Build history of the part. All positions in model axes, mm. A direction names the side the tool comes from. Coordinates: 2 decimals unless noted, no trailing zeros. Order: outer loops, then holes, each group sorted by start corner. A loop starts at its lowest first (then second) coordinate and runs counter-clockwise, first axis right, second up. Notation, with made-up numbers: (-33.75, 41) - (-27.75, 41) arc R17 cw to (-27.75, 62) - close; hole circle Ø9 at (-4.75, -8.5). An arc over 180 degrees is marked (long way). Write each question's results on one line, items separated by ' | '.
from build123d import *

# Parameters (mm, degrees)
SKETCH2_R           = 4.25
SKETCH2_R_2         = 4
BOSS_EXTRUDE1_DEPTH = 15
FILLET1_R           = 1.5


with BuildPart() as part:
    # Sketch2 → Boss-Extrude1 (new body)
    with BuildSketch(Plane.XY):
        with BuildLine():
            Line((0, -35), (26, -35))
            Line((26, -35), (26, -25))
            Line((26, -25), (18, -25))
            Line((18, -25), (18, 0))
            Line((18, 0), (0, 0))
            Line((0, 0), (-18.303795088, -24.696911327))
            Line((-18.303795088, -24.696911327), (-28.121591697, -31.596974351))
            ThreePointArc((-28.121591697, -31.596974351), (-29.945175188, -42.045636622), (-19.496512917, -43.869220113))
            Line((-19.496512917, -43.869220113), (-9.678716308, -36.969157088))
            Line((-9.678716308, -36.969157088), (0, -35))
        make_face()
        with Locations((9, -12.5)):
            Circle(SKETCH2_R, mode=Mode.SUBTRACT)
        with Locations((-23.809052307, -37.733097232)):
            Circle(SKETCH2_R_2, mode=Mode.SUBTRACT)
    extrude(amount=BOSS_EXTRUDE1_DEPTH)

    # Fillet1
    fillet1_edges = [part.edges().sort_by_distance(p)[0] for p in [
        (0, 0, 7.5),
    ]]
    fillet(fillet1_edges, radius=FILLET1_R)


solid = part.part
1. Band-saw the part on C-C on z = 10.5. Give the cut face in (x, y), then the cut area to 3 significant figures.
Solved:
outline: (-28.12, -31.6) arc R7.5 ccw to (-19.5, -43.87) - (-9.68, -36.97) - (0, -35) - (26, -35) - (26, -25) - (18, -25) - (18, 0) - (0.76, 0) arc R1.5 ccw to (-0.45, -0.61) - (-18.3, -24.7) - close; hole circle Ø8 at (-23.81, -37.73); hole circle Ø8.5 at (9, -12.5) | area: 1,260 mm2
2. Two-plate mould, pull along X, no slides. Class faces 4 (the face through (18, -13, 7)), 5 (the face through (-24.676, -41.638, 7.395)), 6 (the face through (5.63, -15.09, 7.4)), 7 (the face through (0.089, -0.156, 7.605)): +X half, -X half, draft (parallel to the pull), parting line (faces both ways), or undercut.
Solved:
face 4: +X half | face 5: undercut | face 6: undercut | face 7: -X half
3. Probe line 1 (Y direction, x = 9, z = 9.25); line 2 (Y direction, x = -23, z = 7.75); line 3 (Y direction, x = 22, z = 5.5). List the from-to ranges inside material, lowest first.
Solved:
line 1: y = -35 to -16.75, -8.25 to 0 | line 2: y = -45.19 to -41.65, -33.82 to -28 | line 3: y = -35 to -25
4. Band-saw the part on D-D on x = 21. Give the cut face in (y, z).
Solved:
outline: (-35, 0) - (-25, 0) - (-25, 15) - (-35, 15) - close
5. Band-saw the part on B-B on y = -41. Give the cut face in (x, z).
Solved:
outline: (-30.56, 0) - (-26.12, 0) - (-26.12, 15) - (-30.56, 15) - close; (-21.5, 0) - (-15.41, 0) - (-15.41, 15) - (-21.5, 15) - close
6. Band-saw the part on A-A on x = 9. Give the cut face in (y, z), then the cut area to 4 significant figures.
Solved:
outline: (-35, 0) - (-16.75, 0) - (-16.75, 15) - (-35, 15) - close; (-8.25, 0) - (0, 0) - (0, 15) - (-8.25, 15) - close | area: 397.5 mm2
7. Tool access for faces 1 (the face through (22, -25, 7)), 2 (the face through (9, 0, 7)), 3 (the face through (13, -35, 7)): list every direction of +Z, -Z, +X, -X, +Y, -Y with a clear straight run to the whole face (end or side of a thin tool).
Solved:
face 1: +Z, -Z, +X, +Y | face 2: +Z, -Z, +X, -X, +Y | face 3: +Z, -Z, +X, -Y
8. Drop flat-ended pins along their axis: pin 1 Ø9 at (x, z) = (21.5, 7) entering from +Y; pin 2 Ø4 at (x, z) = (-25, 12) entering from +Y; pin 3 Ø3 at (y, z) = (-16, 6) entering from -X; pin 4 Ø1.5 at (y, z) = (-14.5, 10.5) entering from +X. Give the stop position or say it passes through.
Solved:
pin 1: stops at y = 0 | pin 2: stops at y = -28 | pin 3: stops at x = -12.97 | pin 4: stops at x = 18
